```python
from build123d import *

# Parameters (mm, degrees)
ESQUISSE1_R             = 2
BOSS_EXTRU_1_DEPTH      = 3
ESQUISSE2_W             = 75
ESQUISSE2_H             = 70
ENL_V_MAT_EXTRU_1_DEPTH = 3
ESQUISSE3_R             = 3
ENL_V_MAT_EXTRU_2_DEPTH = 10


with BuildPart() as part:
    # Esquisse1 → Boss.-Extru.1 (new body)
    with BuildSketch(Plane.XY):
        with BuildLine():
            Line((10, 0), (99, 0))
            Line((99, 0), (99, -36))
            ThreePointArc((99, -36), (135, -72), (171, -36))
            Line((171, -36), (171, 0))
            Line((171, 0), (260, 0))
            ThreePointArc((260, 0), (267.071067812, -2.928932188), (270, -10))
            Line((270, -10), (270, -140))
            ThreePointArc((270, -140), (267.071067812, -147.071067812), (260, -150))
            Line((260, -150), (10, -150))
            ThreePointArc((10, -150), (2.928932188, -147.071067812), (0, -140))
            Line((0, -140), (0, -10))
            ThreePointArc((0, -10), (2.928932188, -2.928932188), (10, 0))
        make_face()
        with Locations((109.4, -121.789429788)):
            Circle(ESQUISSE1_R, mode=Mode.SUBTRACT)
        with Locations((109.4, -86.789429788)):
            Circle(ESQUISSE1_R, mode=Mode.SUBTRACT)
        with Locations((79, -121.789429788)):
            Circle(ESQUISSE1_R, mode=Mode.SUBTRACT)
        with Locations((79, -86.789429788)):
            Circle(ESQUISSE1_R, mode=Mode.SUBTRACT)
        with Locations((162.4, -121.789429788)):
            Circle(ESQUISSE1_R, mode=Mode.SUBTRACT)
        with Locations((162.4, -86.789429788)):
            Circle(ESQUISSE1_R, mode=Mode.SUBTRACT)
        with Locations((191, -121.789429788)):
            Circle(ESQUISSE1_R, mode=Mode.SUBTRACT)
        with Locations((191, -86.789429788)):
            Circle(ESQUISSE1_R, mode=Mode.SUBTRACT)
        with Locations((35.4, -16.191238784)):
            Circle(ESQUISSE1_R, mode=Mode.SUBTRACT)
        with Locations((35.4, -54.191238784)):
            Circle(ESQUISSE1_R, mode=Mode.SUBTRACT)
        with Locations((232.6, -16.191238784)):
            Circle(ESQUISSE1_R, mode=Mode.SUBTRACT)
        with Locations((232.6, -54.191238784)):
            Circle(ESQUISSE1_R, mode=Mode.SUBTRACT)
    extrude(amount=BOSS_EXTRU_1_DEPTH)

    # Esquisse2 → Enlèv. mat.-Extru.1 (cut)
    with BuildSketch(Plane.XY.offset(3)):
        with Locations((37.5, -105)):
            Rectangle(ESQUISSE2_W, ESQUISSE2_H)
        with Locations((232.5, -105)):
            Rectangle(ESQUISSE2_W, ESQUISSE2_H)
    extrude(amount=-ENL_V_MAT_EXTRU_1_DEPTH, mode=Mode.SUBTRACT)

    # Esquisse3 → Enlèv. mat.-Extru.2 (cut)
    with BuildSketch(Plane.XY.offset(3)):
        with Locations((10, -10)):
            Circle(ESQUISSE3_R)
        with Locations((260, -10)):
            Circle(ESQUISSE3_R)
        with Locations((260, -145)):
            Circle(ESQUISSE3_R)
        with Locations((10, -145)):
            Circle(ESQUISSE3_R)
    extrude(amount=-ENL_V_MAT_EXTRU_2_DEPTH, mode=Mode.SUBTRACT)


solid = part.part
```
For this review, take the finished solid that the model builds, in its own axes (mm). Give positions to 0.01 mm unless a question says otherwise; leave off trailing zeros. Write each loop counter-clockwise with the first axis right and the second up, starting at its lowest first coordinate (ties: lowest second). Pieces come first, ordered by that corner, then holes.
Item 1: Wall thickness on probe 1 along Y at (x, z) = (232.6, 1.8); probe 2 along Y at (x, z) = (162.5, 2.5); probe 3 along X at (y, z) = (-37.5, 1.9): over which ranges is each line inside the solid? List them lowest first.
Item 2: Take a section at A-A (y = -32). Give the boundary of the cut face in (x, z), and give its area (3 significant figures).
Item 3: The part is to be moulded in two halves that separate along Y. For faces 1 (the face through (137, -74, 0)), 2 (the face through (2.85, -3.01, 1.48)), 3 (the face through (257, -10, 2)), 4 (the face through (11.61, -142.47, 1.52)), say which applies: +Y half, -Y half, draft (parallel to the pull), parting line (faces both ways), or undercut.
Item 4: Take a section at D-D (x = 135). Give the boundary of the cut face in (y, z), and give its area (3 significant figures).
Item 5: Take a section at C-C (z = 1.95). Give the number of separate pieces and of enclosed holes in the cut face, and give its area (3 significant figures).
Item 6: Take a section at B-B (x = 210). Give the boundary of the cut face in (y, z), and give its area (3 significant figures).
Item 7: Insertion check: P1, Ø5, axis at x = 260, y = -145, coming from the +Z side; P2, Ø1.5, axis at y = -71, z = 1.5, coming from the -X side. Each pin has a flat end and moves straight along its axis. Give the tip position at first contact, or say it passes through.
Established:
1. probe 1: y = -150 to -140, -70 to -56.19, -52.19 to -18.19, -14.19 to 0
1. probe 2: y = -150 to -123.79, -119.79 to -88.79, -84.79 to -59.23
1. probe 3: x = 0 to 99.03, 170.97 to 270
2. outline: (0, 0) - (99, 0) - (99, 3) - (0, 3) - close; (171, 0) - (270, 0) - (270, 3) - (171, 3) - close
2. area: 594 mm2
3. face 1: draft
3. face 2: +Y half
3. face 3: undercut
3. face 4: undercut
4. outline: (-150, 0) - (-72, 0) - (-72, 3) - (-150, 3) - close
4. area: 234 mm2
5. separate pieces: 1
5. enclosed holes: 16
5. area: 25,000 mm2
6. outline: (-150, 0) - (-140, 0) - (-140, 3) - (-150, 3) - close; (-70, 0) - (0, 0) - (0, 3) - (-70, 3) - close
6. area: 240 mm2
7. P1: passes through
7. P2: stops at x = 75
